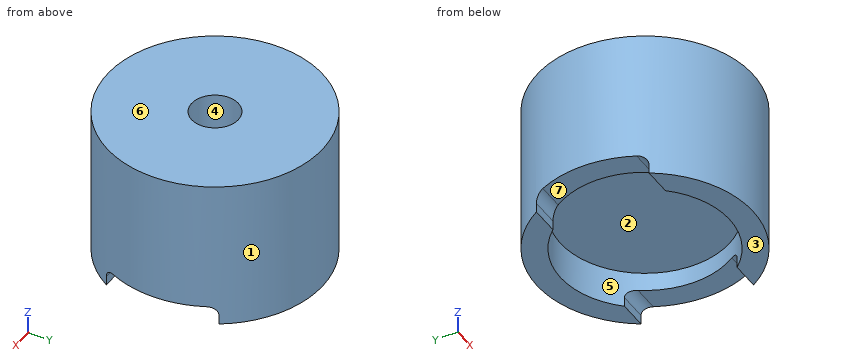
from build123d import *

# Parameters (mm, degrees)
SKIZZE1_R                       = 5.75
AUFSATZ_LINEAR_AUSTRAGEN1_DEPTH = 8
SKIZZE2_R                       = 4.5
SCHNITT_LINEAR_AUSTRAGEN1_DEPTH = 1
SKIZZE3_W                       = 13.35916622
SKIZZE3_H                       = 6
SCHNITT_LINEAR_AUSTRAGEN2_DEPTH = 1
VERRUNDUNG1_R                   = 0.5
SKIZZE4_R                       = 1.25
SCHNITT_LINEAR_AUSTRAGEN3_DEPTH = 3
SKIZZE5_R                       = 4.5
SCHNITT_LINEAR_AUSTRAGEN4_DEPTH = 1


with BuildPart() as part:
    # Skizze1 → Aufsatz-Linear austragen1 (new body)
    with BuildSketch(Plane(origin=(0, 0, 0), x_dir=(0, 1, 0), z_dir=(0, 0, 1))):
        with Locations(Location((0, 0, 0), (0, 0, 270))):
            Circle(SKIZZE1_R)
    extrude(amount=AUFSATZ_LINEAR_AUSTRAGEN1_DEPTH)

    # Skizze2 → Schnitt-Linear austragen1 (cut)
    with BuildSketch(Plane(origin=(0, 0, 0), x_dir=(1, 0, 0), z_dir=(0, 0, -1))):
        with Locations(Location((0, 0, 0), (0, 0, 180))):
            Circle(SKIZZE2_R)
    extrude(amount=-SCHNITT_LINEAR_AUSTRAGEN1_DEPTH, mode=Mode.SUBTRACT)

    # Skizze3 → Schnitt-Linear austragen2 (cut)
    with BuildSketch(Plane(origin=(0, 0, 0), x_dir=(1, 0, 0), z_dir=(0, 0, -1))):
        Rectangle(SKIZZE3_W, SKIZZE3_H)
    extrude(amount=-SCHNITT_LINEAR_AUSTRAGEN2_DEPTH, mode=Mode.SUBTRACT)

    # Verrundung1
    verrundung1_edges = [part.edges().sort_by_distance(p)[0] for p in [
        (4.129728092, 3, 1),
        (-4.129728092, 3, 1),
        (-4.129728092, -3, 1),
        (4.129728092, -3, 1),
    ]]
    fillet(verrundung1_edges, radius=VERRUNDUNG1_R)

    # Skizze4 → Schnitt-Linear austragen3 (cut)
    with BuildSketch(Plane.XY.offset(8)):
        Circle(SKIZZE4_R)
    extrude(amount=-SCHNITT_LINEAR_AUSTRAGEN3_DEPTH, mode=Mode.SUBTRACT)

    # Skizze5 → Schnitt-Linear austragen4 (cut)
    with BuildSketch(Plane(origin=(0, 0, 1), x_dir=(1, 0, 0), z_dir=(0, 0, -1))):
        with Locations(Location((0, 0, 0), (0, 0, 180))):
            Circle(SKIZZE5_R)
    extrude(amount=-SCHNITT_LINEAR_AUSTRAGEN4_DEPTH, mode=Mode.SUBTRACT)


solid = part.part
Geometry check sheet. Reference: the model listing, model coordinates, mm. Face numbers are marked on the shaded views. A direction names the side the tool comes from. Round coordinates to 2 decimals unless told otherwise and drop trailing zeros. Loops run counter-clockwise (first coordinate to the right, second up) from the corner with the lowest first, then second, coordinate; pieces in that order, holes last. Notation, with made-up numbers: (16.25, 65) - (23.25, 65) arc R10 cw to (23.25, 82) - close; hole circle Ø11 at (77, 79.25). An arc over 180 degrees is marked (long way). One line per question, with ' | ' between items. Start each with the question number.
1. Cross-section at C-C on z = 6. Record the cut outline in (x, y).
2. Depth check by flat-ended pin: pin 1 (1.5 mm diameter, centred on x = -3.5, z = 5.5, fed in from -Y); pin 2 (1 mm diameter, centred on y = -4, z = 1.5, fed in from -X); pin 3 (2 mm diameter, centred on x = 5, y = -1, fed in from -Z). Enter the tip coordinate at first touch or a pass-through.
3. Scan lines: line 1 (Y direction, x = 0, z = 1.2); line 2 (Y direction, x = 0, z = 7.05); line 3 (Y direction, x = 2.5, z = 3). Record each from-to range of solid material in increasing order. Write a range as [from, to].
4. Cross-section at D-D on z = 2.25. Record the cut outline in (x, y).
5. Tool access check on the marked faces 4, 5, 6 and 7. Record the directions out of +Z, -Z, +X, -X, +Y, -Y that give a thin tool (end or side, any length) a straight path to the whole face; none if there is none.
6. Cross-section at A-A on x = 0. Record the cut outline in (y, z).
7. Draft check along Y on the marked faces 1, 2 and 3. Enter one of: released by +Y, released by -Y, zero draft, split by the parting line, or undercut.
8. Cross-section at B-B on y = 0. Record the cut outline in (x, z).
Taken from the geometry:
1) outline: circle Ø11.5 at (0, 0); hole circle Ø2.5 at (0, 0)
2) pin 1: y = -5.05 | pin 2: x = -4.56 | pin 3: z = 1
3) line 1: [-5.75, -4.5], [4.5, 5.75] | line 2: [-5.75, -1.25], [1.25, 5.75] | line 3: [-5.18, 5.18]
4) outline: circle Ø11.5 at (0, 0)
5) face 4: +Z | face 5: -Z | face 6: +Z, +X, -X, +Y, -Y | face 7: -Z, +X, -X
6) outline: (-5.75, 0) - (-4.5, 0) - (-4.5, 2) - (4.5, 2) - (4.5, 0) - (5.75, 0) - (5.75, 8) - (1.25, 8) - (1.25, 5) - (-1.25, 5) - (-1.25, 8) - (-5.75, 8) - close
7) face 1: split by the parting line | face 2: undercut | face 3: zero draft
8) outline: (-5.75, 1) - (-4.5, 1) - (-4.5, 2) - (4.5, 2) - (4.5, 1) - (5.75, 1) - (5.75, 8) - (1.25, 8) - (1.25, 5) - (-1.25, 5) - (-1.25, 8) - (-5.75, 8) - close
